Here's how the part is built. I have some questions about the finished solid (model axes, mm). Face numbers are marked on the shaded views. A direction names the side the tool comes from. Give positions to 0.01 mm unless a question says otherwise; leave off trailing zeros. Order: outer loops, then holes, each group sorted by start corner. A loop starts at its lowest first (then second) coordinate and runs counter-clockwise, first axis right, second up. Notation, with made-up numbers: M 86,13 L 141,13 A29 ccw 141,44 Z; hole C 84.25,46 d11. An arc over 180 degrees is marked long. Use one line per item in the form item = value.
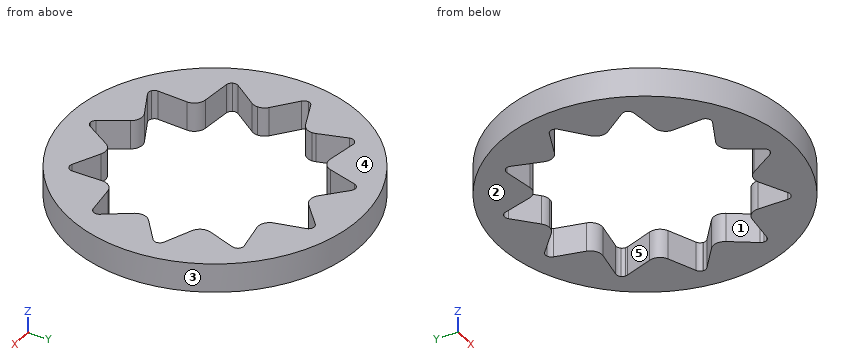
from build123d import *

# Parameters (mm, degrees)
F0_R     = 15.875
F1_DEPTH = 3.175


with BuildPart() as f1:
    # F0 (on Top) → F1 (new body)
    with BuildSketch(Plane.XY):
        Circle(F0_R)
        with BuildLine():
            ThreePointArc((0, 13.49375), (1.920361, 13.356403), (3.801629, 12.947158))
            ThreePointArc((3.801629, 12.947158), (7.295272, 11.351665), (10.197896, 8.836527))
            ThreePointArc((10.197896, 8.836527), (12.274347, 5.605506), (13.356403, 1.920361))
            ThreePointArc((13.356403, 1.920361), (13.459369, 0.962633), (13.49375, 0))
            ThreePointArc((13.49375, 0), (13.185376, -2.868303), (12.274347, -5.605506))
            ThreePointArc((12.274347, -5.605506), (10.197896, -8.836527), (7.295272, -11.351665))
            ThreePointArc((7.295272, -11.351665), (3.801629, -12.947158), (0, -13.49375))
            ThreePointArc((0, -13.49375), (-3.801629, -12.947158), (-7.295272, -11.351665))
            ThreePointArc((-7.295272, -11.351665), (-10.197896, -8.836527), (-12.274347, -5.605506))
            ThreePointArc((-12.274347, -5.605506), (-13.356403, -1.920361), (-13.356403, 1.920361))
            ThreePointArc((-13.356403, 1.920361), (-12.274347, 5.605506), (-10.197896, 8.836527))
            ThreePointArc((-10.197896, 8.836527), (-7.295272, 11.351665), (-3.801629, 12.947158))
            ThreePointArc((-3.801629, 12.947158), (-1.920361, 13.356403), (0, 13.49375))
        make_face(mode=Mode.SUBTRACT)
        with BuildLine():
            ThreePointArc((-4.237237, 12.497892), (-4.078617, 12.77991), (-3.801629, 12.947158))
            ThreePointArc((-3.801629, 12.947158), (-7.295272, 11.351665), (-10.197896, 8.836527))
            ThreePointArc((-10.197896, 8.836527), (-9.930697, 9.019007), (-9.608271, 9.046139))
            Line((-9.608271, 9.046139), (-6.484799, 8.49818))
            ThreePointArc((-6.484799, 8.49818), (-7.082113, 10.721599), (-4.995351, 9.749077))
            ThreePointArc((-4.995351, 9.749077), (-5.005639, 9.587758), (-5.036334, 9.429053))
            Line((-5.036334, 9.429053), (-4.237237, 12.497892))
        make_face()
        with BuildLine():
            ThreePointArc((-6.484799, 8.49818), (-5.578737, 8.680685), (-5.036334, 9.429053))
            ThreePointArc((-5.036334, 9.429053), (-5.005639, 9.587758), (-4.995351, 9.749077))
            ThreePointArc((-4.995351, 9.749077), (-7.082113, 10.721599), (-6.484799, 8.49818))
        make_face()
        with BuildLine():
            ThreePointArc((-13.128695, 1.337485), (-13.319334, 1.598926), (-13.356403, 1.920361))
            ThreePointArc((-13.356403, 1.920361), (-13.356403, -1.920361), (-12.274347, -5.605506))
            ThreePointArc((-12.274347, -5.605506), (-12.329338, -5.286648), (-12.220077, -4.982089))
            Line((-12.220077, -4.982089), (-10.4241, -2.368509))
            ThreePointArc((-10.4241, -2.368509), (-12.727866, -1.829991), (-10.669136, -0.66424))
            Line((-10.669136, -0.66424), (-13.128695, 1.337485))
        make_face()
        with BuildLine():
            ThreePointArc((-10.200793, -1.649251), (-10.32384, -1.103909), (-10.669136, -0.66424))
            ThreePointArc((-10.669136, -0.66424), (-12.727866, -1.829991), (-10.4241, -2.368509))
            ThreePointArc((-10.4241, -2.368509), (-10.257904, -2.025814), (-10.200793, -1.649251))
        make_face()
        with BuildLine():
            ThreePointArc((-10.321462, 8.223073), (-10.340492, 8.546078), (-10.197896, 8.836527))
            ThreePointArc((-10.197896, 8.836527), (-12.274347, 5.605506), (-13.356403, 1.920361))
            ThreePointArc((-13.356403, 1.920361), (-13.230277, 2.218332), (-12.973704, 2.415473))
            Line((-12.973704, 2.415473), (-10.049823, 3.643177))
            ThreePointArc((-10.049823, 3.643177), (-11.69673, 5.341718), (-9.334564, 5.209376))
            Line((-9.334564, 5.209376), (-10.321462, 8.223073))
        make_face()
        with BuildLine():
            ThreePointArc((-9.271498, 4.814141), (-9.287363, 5.014259), (-9.334564, 5.209376))
            ThreePointArc((-9.334564, 5.209376), (-11.69673, 5.341718), (-10.049823, 3.643177))
            ThreePointArc((-10.049823, 3.643177), (-9.483829, 4.111121), (-9.271498, 4.814141))
        make_face()
        with BuildLine():
            Line((0, 12.85875), (0, 13.49375))
            ThreePointArc((0, 13.49375), (-1.920361, 13.356403), (-3.801629, 12.947158))
            ThreePointArc((-3.801629, 12.947158), (-3.47819, 12.956212), (-3.19228, 12.80472))
            Line((-3.19228, 12.80472), (-0.860897, 10.655071))
            ThreePointArc((-0.860897, 10.655071), (-1.182935, 12.05088), (0, 12.85875))
        make_face()
        with BuildLine():
            ThreePointArc((1.27, 11.58875), (0.898026, 12.486776), (0, 12.85875))
            Line((0, 12.85875), (0, 10.31875))
            ThreePointArc((0, 10.31875), (0.46213, 10.405815), (0.860897, 10.655071))
            ThreePointArc((0.860897, 10.655071), (1.163237, 11.079064), (1.27, 11.58875))
        make_face()
        with BuildLine():
            ThreePointArc((3.19228, 12.80472), (3.47819, 12.956212), (3.801629, 12.947158))
            ThreePointArc((3.801629, 12.947158), (1.920361, 13.356403), (0, 13.49375))
            Line((0, 13.49375), (0, 12.85875))
            ThreePointArc((0, 12.85875), (0.898026, 12.486776), (1.27, 11.58875))
            ThreePointArc((1.27, 11.58875), (1.163237, 11.079064), (0.860897, 10.655071))
            Line((0.860897, 10.655071), (3.19228, 12.80472))
        make_face()
        with BuildLine():
            Line((0, 10.31875), (0, 12.85875))
            ThreePointArc((0, 12.85875), (-1.182935, 12.05088), (-0.860897, 10.655071))
            ThreePointArc((-0.860897, 10.655071), (-0.46213, 10.405815), (0, 10.31875))
        make_face()
        with BuildLine():
            ThreePointArc((10.197896, 8.836527), (7.295272, 11.351665), (3.801629, 12.947158))
            ThreePointArc((3.801629, 12.947158), (4.078617, 12.77991), (4.237237, 12.497892))
            Line((4.237237, 12.497892), (5.036334, 9.429053))
            ThreePointArc((5.036334, 9.429053), (6.104032, 11.00879), (7.535351, 9.749077))
            ThreePointArc((7.535351, 9.749077), (7.237874, 8.932315), (6.484799, 8.49818))
            Line((6.484799, 8.49818), (9.608271, 9.046139))
            ThreePointArc((9.608271, 9.046139), (9.930697, 9.019007), (10.197896, 8.836527))
        make_face()
        with BuildLine():
            ThreePointArc((7.535351, 9.749077), (6.104032, 11.00879), (5.036334, 9.429053))
            ThreePointArc((5.036334, 9.429053), (5.578737, 8.680685), (6.484799, 8.49818))
            ThreePointArc((6.484799, 8.49818), (7.237874, 8.932315), (7.535351, 9.749077))
        make_face()
        with BuildLine():
            ThreePointArc((13.356403, 1.920361), (12.274347, 5.605506), (10.197896, 8.836527))
            ThreePointArc((10.197896, 8.836527), (10.312958, 8.6426), (10.352995, 8.420691))
            ThreePointArc((10.352995, 8.420691), (10.345062, 8.320632), (10.321462, 8.223073))
            Line((10.321462, 8.223073), (9.334564, 5.209376))
            ThreePointArc((9.334564, 5.209376), (10.741616, 6.068275), (11.811498, 4.814141))
            ThreePointArc((11.811498, 4.814141), (11.244518, 3.756472), (10.049823, 3.643177))
            Line((10.049823, 3.643177), (12.973704, 2.415473))
            ThreePointArc((12.973704, 2.415473), (13.230277, 2.218332), (13.356403, 1.920361))
        make_face()
        with BuildLine():
            ThreePointArc((9.334564, 5.209376), (9.386265, 4.286564), (10.049823, 3.643177))
            ThreePointArc((10.049823, 3.643177), (11.244518, 3.756472), (11.811498, 4.814141))
            ThreePointArc((11.811498, 4.814141), (10.741616, 6.068275), (9.334564, 5.209376))
        make_face()
        with BuildLine():
            ThreePointArc((13.49375, 0), (13.459369, 0.962633), (13.356403, 1.920361))
            ThreePointArc((13.356403, 1.920361), (13.361249, 1.875291), (13.362866, 1.829991))
            ThreePointArc((13.362866, 1.829991), (13.301343, 1.55732), (13.128695, 1.337486))
            Line((13.128695, 1.337486), (10.669136, -0.66424))
            ThreePointArc((10.669136, -0.66424), (12.016135, -0.502298), (12.740793, -1.649251))
            ThreePointArc((12.740793, -1.649251), (11.847356, -2.86214), (10.4241, -2.368509))
            Line((10.4241, -2.368509), (12.220077, -4.982089))
            ThreePointArc((12.220077, -4.982089), (12.303175, -5.153436), (12.33173, -5.341718))
            ThreePointArc((12.33173, -5.341718), (12.317219, -5.476697), (12.274347, -5.605506))
            ThreePointArc((12.274347, -5.605506), (13.185376, -2.868303), (13.49375, 0))
        make_face()
        with BuildLine():
            ThreePointArc((12.740793, -1.649251), (12.016135, -0.502298), (10.669136, -0.66424))
            ThreePointArc((10.669136, -0.66424), (10.21372, -1.468511), (10.4241, -2.368509))
            ThreePointArc((10.4241, -2.368509), (11.847356, -2.86214), (12.740793, -1.649251))
        make_face()
        with BuildLine():
            ThreePointArc((7.295272, -11.351665), (10.197896, -8.836527), (12.274347, -5.605506))
            ThreePointArc((12.274347, -5.605506), (12.069382, -5.855873), (11.76766, -5.972744))
            Line((11.76766, -5.972744), (8.616333, -6.326965))
            ThreePointArc((8.616333, -6.326965), (9.604579, -6.642164), (10.028193, -7.589017))
            ThreePointArc((10.028193, -7.589017), (8.777792, -8.858866), (7.488798, -7.628211))
            Line((7.488798, -7.628211), (7.586663, -10.797872))
            ThreePointArc((7.586663, -10.797872), (7.58689, -10.807669), (7.586965, -10.817469))
            ThreePointArc((7.586965, -10.817469), (7.509291, -11.121792), (7.295272, -11.351665))
        make_face()
        with BuildLine():
            ThreePointArc((10.028193, -7.589017), (9.604579, -6.642164), (8.616333, -6.326965))
            ThreePointArc((8.616333, -6.326965), (7.798391, -6.757344), (7.488798, -7.628211))
            ThreePointArc((7.488798, -7.628211), (8.777792, -8.858866), (10.028193, -7.589017))
        make_face()
        with BuildLine():
            ThreePointArc((0, -13.49375), (3.801629, -12.947158), (7.295272, -11.351665))
            ThreePointArc((7.295272, -11.351665), (6.987486, -11.451475), (6.670477, -11.386669))
            Line((6.670477, -11.386669), (3.827905, -9.980923))
            ThreePointArc((3.827905, -9.980923), (4.343789, -10.44928), (4.534928, -11.119324))
            ThreePointArc((4.534928, -11.119324), (2.925975, -12.343257), (2.175856, -10.466009))
            Line((2.175856, -10.466009), (0.544536, -13.185408))
            ThreePointArc((0.544536, -13.185408), (0.312888, -13.411313), (0, -13.49375))
        make_face()
        with BuildLine():
            ThreePointArc((4.534928, -11.119324), (4.343789, -10.44928), (3.827905, -9.980923))
            ThreePointArc((3.827905, -9.980923), (2.907128, -9.900768), (2.175856, -10.466009))
            ThreePointArc((2.175856, -10.466009), (2.925975, -12.343257), (4.534928, -11.119324))
        make_face()
        with BuildLine():
            ThreePointArc((-6.670476, -11.386669), (-6.987486, -11.451475), (-7.295272, -11.351665))
            ThreePointArc((-7.295272, -11.351665), (-3.801629, -12.947158), (0, -13.49375))
            ThreePointArc((0, -13.49375), (-0.312888, -13.411313), (-0.544536, -13.185408))
            Line((-0.544536, -13.185408), (-2.175856, -10.466009))
            ThreePointArc((-2.175856, -10.466009), (-2.040996, -10.780371), (-1.994928, -11.119324))
            ThreePointArc((-1.994928, -11.119324), (-3.934973, -12.198185), (-3.827905, -9.980923))
            Line((-3.827905, -9.980923), (-6.670476, -11.386669))
        make_face()
        with BuildLine():
            ThreePointArc((-2.175856, -10.466009), (-2.907128, -9.900768), (-3.827905, -9.980923))
            ThreePointArc((-3.827905, -9.980923), (-3.934973, -12.198185), (-1.994928, -11.119324))
            ThreePointArc((-1.994928, -11.119324), (-2.040996, -10.780371), (-2.175856, -10.466009))
        make_face()
        with BuildLine():
            ThreePointArc((-11.76766, -5.972744), (-12.069382, -5.855874), (-12.274347, -5.605506))
            ThreePointArc((-12.274347, -5.605506), (-10.197896, -8.836527), (-7.295272, -11.351665))
            ThreePointArc((-7.295272, -11.351665), (-7.513921, -11.113155), (-7.586663, -10.797872))
            Line((-7.586663, -10.797872), (-7.488798, -7.628211))
            ThreePointArc((-7.488798, -7.628211), (-9.717995, -8.42069), (-8.616333, -6.326965))
            Line((-8.616333, -6.326965), (-11.76766, -5.972744))
        make_face()
        with BuildLine():
            ThreePointArc((-7.488193, -7.589017), (-7.81134, -6.742631), (-8.616333, -6.326965))
            ThreePointArc((-8.616333, -6.326965), (-9.717995, -8.42069), (-7.488798, -7.628211))
            ThreePointArc((-7.488798, -7.628211), (-7.488344, -7.608616), (-7.488193, -7.589017))
        make_face()
    extrude(amount=-F1_DEPTH)


solid = f1.part
Q1. I want a section at B-B on y = 0. Write out the boundary of the cut face in (x, z) (3 decimals).
Found:
outline = M -15.875,-3.175 L -11.485,-3.175 L -11.485,0 L -15.875,0 Z; M 11.485,-3.175 L 15.875,-3.175 L 15.875,0 L 11.485,0 Z
Q2. I want a section at C-C on x = 14. Write out the boundary of the cut face in (y, z) (3 decimals), then the cut area to 3 significant figures.
Found:
outline = M -7.484,-3.175 L 7.484,-3.175 L 7.484,0 L -7.484,0 Z
area = 47.5 mm²
Q3. I want a section at A-A on x = 8. Write out the boundary of the cut face in (y, z) (3 decimals).
Found:
outline = M -13.712,-3.175 L -6.57,-3.175 L -6.57,0 L -13.712,0 Z; M 8.764,-3.175 L 13.712,-3.175 L 13.712,0 L 8.764,0 Z
Q4. I need wall thicknesses on L1, parallel to Y at x = -11, z = -2.7; L2, parallel to X at y = -9, z = -2.55; L3, parallel to X at y = -2.5, z = -2.95. Which ranges of each line are inside material? Lowest first, please.
Found:
L1 = -11.45 to -6.06, -3.21 to -0.39, 3.24 to 11.45
L2 = -13.08 to -7.53, 7.53 to 13.08
L3 = -15.68 to -10.51, 10.51 to 15.68
Q5. I'm going to push flat-ended pins straight in: pin 1 Ø1 at (x, z) = (-2, -0.5) entering from +Y; pin 2 Ø1.5 at (y, z) = (3, -0.5) entering from +X. Where does each tip first touch, or does it pass through?
Found:
pin_1 = 15.8
pin_2 = 15.71
Q6. Thinking about a two-plate mould opening in X: for the marked faces 1, 2 and 3, which applies, +X half, -X half, draft (parallel to the pull), parting line (faces both ways), or undercut?
Found:
face_1 = undercut
face_2 = draft
face_3 = parting line
Q7. On a 3-axis mill with a long thin cutter (end or side, diameter ignored), from which of +Z, -Z, +X, -X, +Y, -Y can I reach the whole of each face in a straight line? I mean the marked faces 4 and 5. Say none if no direction works.
Found:
face_4 = +Z, +X, -X, +Y, -Y
face_5 = +Z, -Z
